from build123d import *

# Parameters (mm, degrees)
SALIENTE_EXTRUIR1_DEPTH = 32
CORTAR_EXTRUIR2_DEPTH   = 33
SALIENTE_EXTRUIR2_DEPTH = 0.01
SALIENTE_EXTRUIR3_DEPTH = 0.01
SALIENTE_EXTRUIR5_DEPTH = 0.01
SALIENTE_EXTRUIR6_DEPTH = 0.01


with BuildPart() as part:
    # Croquis1 → Saliente-Extruir1 (new body)
    with BuildSketch(Plane.XY):
        Polygon((-23.483096056, 8.186360271), (-55.483096056, 8.189793686), (-55.483096056, 18.141275036), (-23.483096056, 18.141275036), align=None)
        Polygon((-23.483096056, 8.186360271), (-35.959662641, -4.290206314), (-43.003096056, -4.290206314), (-55.483096056, 8.189793686), align=None)
    extrude(amount=SALIENTE_EXTRUIR1_DEPTH)

    # Croquis2 → Cortar-Extruir2 (cut)
    with BuildSketch(Plane(origin=(-23.483096056, 0, 0), x_dir=(0, 0, -1), z_dir=(1, 0, 0))):
        Polygon((-12.476566586, -4.290206314), (0, -4.290206314), (0, 8.186360271), align=None)
        Polygon((-32, -4.290206314), (-32, 8.186360271), (-19.523433414, -4.290206314), align=None)
    extrude(amount=-CORTAR_EXTRUIR2_DEPTH, mode=Mode.SUBTRACT)

    # Croquis3 → Saliente-Extruir2 (add)
    with BuildSketch(Plane(origin=(0, 4.093180136, 4.093180136), x_dir=(-1, 0, 0), z_dir=(0, -0.707106781, -0.707106781))):
        with BuildLine():
            Line((28.08600417, 2.901010434), (50.876754527, 2.901010434))
            ThreePointArc((50.876754527, 2.901010434), (39.481379348, -8.494364744), (28.08600417, 2.901010434))
        make_face()
    extrude(amount=SALIENTE_EXTRUIR2_DEPTH)

    # Croquis4 → Saliente-Extruir3 (add)
    with BuildSketch(Plane(origin=(-15.834728163, 15.834728163, 0), x_dir=(-0.707106781, -0.707106781, 0), z_dir=(0.707106781, -0.707106781, 0))):
        with BuildLine():
            Line((13.640847296, -27.43326467), (13.640847296, -4.56673533))
            ThreePointArc((13.640847296, -4.56673533), (25.074111966, -16), (13.640847296, -27.43326467))
        make_face()
    extrude(amount=SALIENTE_EXTRUIR3_DEPTH)

    # Croquis5 → Saliente-Extruir5 (add)
    with BuildSketch(Plane(origin=(0, -11.906819864, 11.906819864), x_dir=(1, 0, 0), z_dir=(0, -0.707106781, 0.707106781))):
        with BuildLine():
            Line((-27.929927847, 25.798759553), (-39.481379348, 25.798759553))
            Line((-39.481379348, 25.798759553), (-51.03283085, 25.798759553))
            ThreePointArc((-51.03283085, 25.798759553), (-39.481379348, 14.247308052), (-27.929927847, 25.798759553))
        make_face()
    extrude(amount=SALIENTE_EXTRUIR5_DEPTH)

    # Croquis6 → Saliente-Extruir6 (add)
    with BuildSketch(Plane(origin=(-23.646651185, -23.646651185, 0), x_dir=(-0.707106781, 0.707106781, 0), z_dir=(-0.707106781, -0.707106781, 0))):
        with BuildLine():
            Line((42.153256878, -4.590405514), (42.153256878, -27.409594486))
            ThreePointArc((42.153256878, -27.409594486), (30.743662392, -16), (42.153256878, -4.590405514))
        make_face()
    extrude(amount=SALIENTE_EXTRUIR6_DEPTH)


solid = part.part
Input: part model. Units: mm. Frame: model coordinates. Round coordinates to 2 decimals unless told otherwise and drop trailing zeros. Order: outer loops, then holes, each group sorted by start corner. A loop starts at its lowest first (then second) coordinate and runs counter-clockwise, first axis right, second up.
1. Pin query (flat end, axial travel): P1, Ø1, axis at x = -50.5, y = 4, coming from the -Z side; P2, Ø1, axis at y = 6.5, z = 8, coming from the -X side; P3, Ø1.5, axis at x = -28.5, z = 25.5, coming from the -Y side; P4, Ø10, axis at x = -51, y = 3.5, coming from the +Z side. Return the tip coordinate at first contact, or that it passes through.
The answers:
P1: stops at z = 3.67
P2: stops at x = -54.29
P3: stops at y = 2.41
P4: stops at z = 32
2. Material intervals for line 1 (Y direction, x = -31.5, z = 2); line 2 (Y direction, x = -53, z = 29); line 3 (X direction, y = 4.25, z = 9), sorted ascending.
The answers:
line 1: y = 6.19 to 18.14
line 2: y = 5.71 to 18.14
line 3: x = -51.56 to -27.41
3. Cut plane C-C, the plane y = 7.25. Output: boundary loops of the cut face in (x, z).
The answers:
outline: (-54.54, 0.94) - (-24.42, 0.94) - (-24.42, 31.06) - (-54.54, 31.06) - close
